Can you work these out from the model? Positions are in its coordinate system, mm. Give positions to 0.01 mm unless a question says otherwise; leave off trailing zeros. Order: outer loops, then holes, each group sorted by start corner. A loop starts at its lowest first (then second) coordinate and runs counter-clockwise, first axis right, second up. Notation, with made-up numbers: (-8, 20.5) - (9, 20.5) arc R6 ccw to (9, 25.5) - close; hole circle Ø3 at (34.5, -22.75). An arc over 180 degrees is marked (long way). Answer as CSV lines item,"result".
```python
from build123d import *

# Parameters (mm, degrees)
SKETCH1_R           = 1.5
BOSS_EXTRUDE1_DEPTH = 5
BOSS_EXTRUDE2_START = -42.7
SKETCH1_2_R         = 1.5
BOSS_EXTRUDE2_DEPTH = 42.7
BOSS_EXTRUDE3_START = -47.7
SKETCH1_4_R         = 1.5
BOSS_EXTRUDE3_DEPTH = 5


with BuildPart() as part:
    # Sketch1 → Boss-Extrude1 (new body)
    with BuildSketch(Plane(origin=(0, 0, 0), x_dir=(1, 0, 0), z_dir=(0, 1, 0))):
        Polygon((0, 0), (0, -15), (15, -15), align=None)
        with Locations(Location((3.8, -10.5, 0), (0, 0, 270))):
            Circle(SKETCH1_R, mode=Mode.SUBTRACT)
    extrude(amount=BOSS_EXTRUDE1_DEPTH)

    # Sketch1_2 → Boss-Extrude2 (add)
    # profile 1 of 2: a face of its own
    with BuildSketch(Plane(origin=(0, 0, 0), x_dir=(1, 0, 0), z_dir=(0, 1, 0)).offset(BOSS_EXTRUDE2_START)):
        Polygon((0, -15), (15, -15), (0, 0), align=None)
        with Locations(Location((3.8, -10.5, 0), (0, 0, 270))):
            Circle(SKETCH1_2_R, mode=Mode.SUBTRACT)
    # profile 2 of 2: a face of its own
    with BuildSketch(Plane(origin=(0, 0, 0), x_dir=(1, 0, 0), z_dir=(0, 1, 0)).offset(BOSS_EXTRUDE2_START)):
        with Locations(Location((3.8, -10.5, 0), (0, 0, 270))):
            Circle(SKETCH1_2_R)
    extrude(amount=BOSS_EXTRUDE2_DEPTH)

    # Sketch1_4 → Boss-Extrude3 (add)
    with BuildSketch(Plane(origin=(0, 0, 0), x_dir=(1, 0, 0), z_dir=(0, 1, 0)).offset(BOSS_EXTRUDE3_START)):
        Polygon((0, -15), (15, -15), (0, 0), align=None)
        with Locations(Location((3.8, -10.5, 0), (0, 0, 270))):
            Circle(SKETCH1_4_R, mode=Mode.SUBTRACT)
    extrude(amount=BOSS_EXTRUDE3_DEPTH)


solid = part.part
```
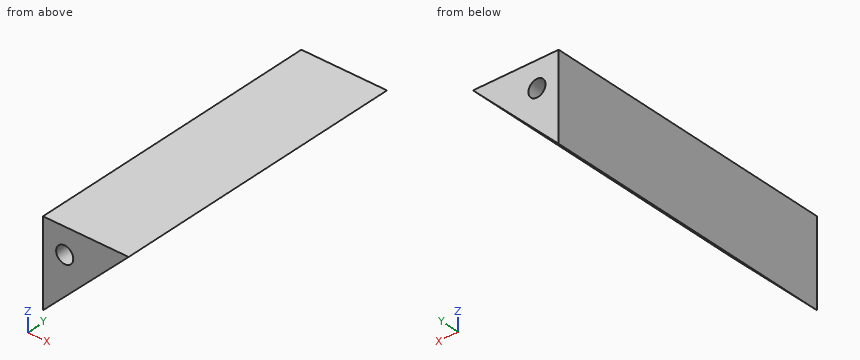
1) I want a section at D-D on z = 1. Write out the boundary of the cut face in (x, y), plus the area to 3 significant figures.
Answer block:
outline,"(0, -47.7) - (1, -47.7) - (1, 5) - (0, 5) - close"
area,"52.7 mm2"
2) I'm going to push flat-ended pins straight in: P1, Ø2, axis at y = -11, z = 12.5, coming from the +X side; P2, Ø1.8, axis at x = 3.8, z = 10.5, coming from the +Y side; P3, Ø0.9, axis at x = 4, z = 10.5, coming from the -Y side. Where does each tip first touch, or does it pass through?
Answer block:
P1,"x = 13.5"
P2,"y = 0"
P3,"y = -42.7"
3) I need wall thicknesses on line 1 along Z through (x, y) = (12, -17); line 2 along X through (y, z) = (1.75, 10.5); line 3 along Z through (x, y) = (9, 3.5). Which ranges of each line are inside material? Lowest first, please. Write a range as [from, to].
Answer block:
line 1,"[12, 15]"
line 2,"[0, 2.3], [5.3, 10.5]"
line 3,"[9, 15]"
4) I want a section at C-C on y = -14.5. Write out the boundary of the cut face in (x, z), plus the area to 4 significant figures.
Answer block:
outline,"(0, 0) - (15, 15) - (0, 15) - close"
area,"112.5 mm2"
5) I want a section at B-B on x = 3.8. Write out the boundary of the cut face in (y, z).
Answer block:
outline,"(-47.7, 3.8) - (5, 3.8) - (5, 9) - (0, 9) - (0, 12) - (5, 12) - (5, 15) - (-47.7, 15) - (-47.7, 12) - (-42.7, 12) - (-42.7, 9) - (-47.7, 9) - close"
6) I want a section at A-A on z = 10.5. Write out the boundary of the cut face in (x, y), plus the area to 3 significant figures.
Answer block:
outline,"(0, -47.7) - (2.3, -47.7) - (2.3, -42.7) - (5.3, -42.7) - (5.3, -47.7) - (10.5, -47.7) - (10.5, 5) - (5.3, 5) - (5.3, 0) - (2.3, 0) - (2.3, 5) - (0, 5) - close"
area,"523 mm2"
